Geometry: see drawing. Coordinates: mm, zero at the bounding-box minimum. Round coordinates to 2 decimals unless told otherwise and drop trailing zeros. Loops run counter-clockwise (first coordinate to the right, second up) from the corner with the lowest first, then second, coordinate; pieces in that order, holes last. Notation, with made-up numbers: M 72,-6 L 89,-6 A23 ccw 89,16 Z; hole C 31,13 d10. An arc over 180 degrees is marked long. Answer as a JSON object with one key per item and string values.
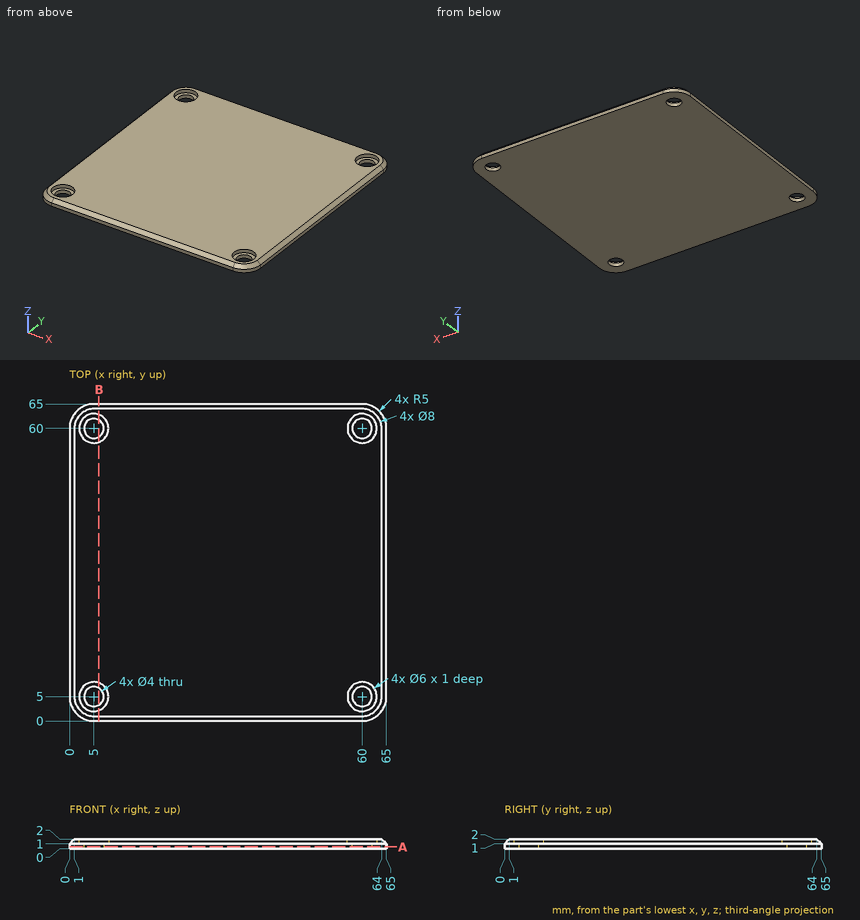
1) Pin query (flat end, axial travel): P1, Ø3.5, axis at x = 5, y = 5, coming from the +Z side; P2, Ø4.5, axis at x = 5, y = 60, coming from the +Z side. Return the tip coordinate at first contact, or that it passes through.
Results:
{"P1": "through", "P2": "z = 1"}
2) Ray query, line 1 (Y direction, x = 57.5, z = 1.65); line 2 (Y direction, x = 59.5, z = 0.25); line 3 (X direction, y = 22, z = 1.6). Return the intervals inside material, ascending.
Results:
{"line 1": "0.65 to 3.34, 6.66 to 58.34, 61.66 to 64.35", "line 2": "0 to 3.06, 6.94 to 58.06, 61.94 to 65", "line 3": "0.6 to 64.4"}
3) Section query B-B (x = 6). Return the cut outline in (y, z).
Results:
{"outline": "M 0,0 L 3.27,0 L 3.27,1 L 2.17,1 L 2.17,2 L 1,2 L 0,1 Z; M 6.73,0 L 58.27,0 L 58.27,1 L 57.17,1 L 57.17,2 L 7.83,2 L 7.83,1 L 6.73,1 Z; M 61.73,0 L 65,0 L 65,1 L 64,2 L 62.83,2 L 62.83,1 L 61.73,1 Z"}
4) Section query A-A (z = 0.4). Return the cut outline in (x, y).
Results:
{"outline": "M 0,5 A5 ccw 5,0 L 60,0 A5 ccw 65,5 L 65,60 A5 ccw 60,65 L 5,65 A5 ccw 0,60 Z; hole C 5,5 d4; hole C 5,60 d4; hole C 60,5 d4; hole C 60,60 d4"}
